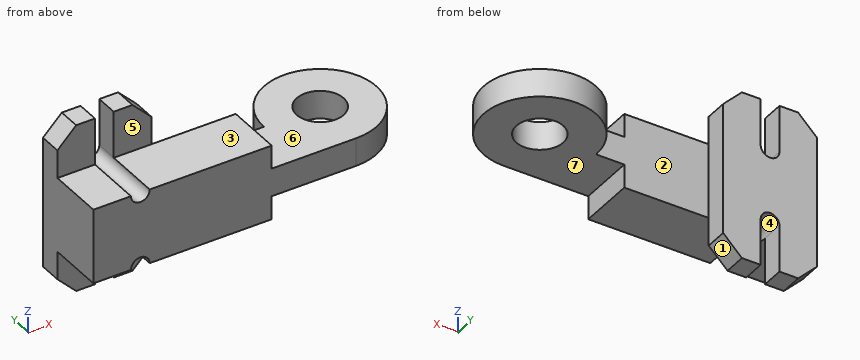
Autodesk Inventor part; units mm, degrees
ref_plane "YZ Plane" through (0, 0, 0) normal (1, 0, 0) x (0, 1, 0)
ref_plane "XZ Plane" through (0, 0, 0) normal (0, 1, 0) x (-1, 0, 0)
ref_plane "XY Plane" through (0, 0, 0) normal (0, 0, 1) x (1, 0, 0)
sketch "Esboço1" plane through (0, 0, 0) normal (0, 0, 1) x (1, 0, 0)
  line L0 (0, 0) -> (95, 0)
  line L1 (95, 0) -> (95, 30)
  line L2 (95, 30) -> (0, 30)
  line L3 (0, 30) -> (0, 0)
  line L4 (0, 30) -> (50, 30)
  line L5 (50, 30) -> (50, 42)
  line L6 (50, 42) -> (0, 42)
  line L7 (0, 42) -> (0, 30)
  line L8 (95, 0) -> (140, 0)
  line L9 (110, 30) -> (95, 30)
  line L10 (95, 30) -> (95, 0)
  arc A0 (140, 0) -> (110, 30) centre (140, 30) ccw
  dimension "d0" = 95
  dimension "d1" = 30
  dimension "d2" = 50
  dimension "d3" = 12
  dimension "d5" = 60
  dimension "d6" = 140
extrude "Extrusão1" add sketch "Esboço1" along normal mid plane 40 contours L3 L2 L1 L0
extrude "Extrusão2" add sketch "Esboço1" along normal mid plane 90 contours L7 L6 L5 L2
extrude "Extrusão3" add sketch "Esboço1" along normal mid plane 15 contours L1 L9 A0 L8
sketch "Esboço2" plane through (0, 0, 7.5) normal (0, 0, 1) x (1, 0, 0)
  arc A0 (140, 0) -> (110, 30) centre (140, 30) ccw
  point P0 (0, 0)
hole "Furo1" at (140, 30, 7.5) direction (0, 0, -1) diameter 25 end through all
sketch "Esboço3" plane through (0, 42, 45) normal (0, 1, 0) x (1, 0, 0)
  line L0 (25, -25) -> (25, 25) construction
  line L1 (50, 0) -> (0, 0)
  line L2 (30, -25) -> (30, 25)
  line L3 (20, 25) -> (20, -25)
  arc A0 (20, -25) -> (30, -25) centre (25, -25) ccw
  arc A1 (30, 25) -> (20, 25) centre (25, 25) ccw
  line L4 (25, 115) -> (25, 65) construction
  line L5 (50, 90) -> (0, 90)
  line L6 (20, 115) -> (20, 65)
  line L7 (30, 65) -> (30, 115)
  arc A2 (30, 115) -> (20, 115) centre (25, 115) ccw
  arc A3 (20, 65) -> (30, 65) centre (25, 65) ccw
  point P0 (0, 45)
  point P1 (25, 0)
  point P2 (25, 90)
  point P3 (20, 0)
  point P4 (30, 0)
  dimension "d20" = 5
  dimension "d21" = 5
  dimension "d22" = 25
  dimension "d23" = 25
extrude "Extrusão4" cut sketch "Esboço3" against normal through all contours L1 L3 A1 L2
extrude "Extrusão5" cut sketch "Esboço3" against normal through all contours L7 A3 L6 L5 | L5 L6 A2 L7
chamfer "Chanfro1" distance 10 angle 45 1 edges at (0, 36, 45) measured on face at (0, 10, 6.6667)
chamfer "Chanfro2" distance 10 angle 45 1 edges at (50, 36, 45) measured on face at (50, 38, -6.6667)
chamfer "Chanfro3" distance 10 angle 45 1 edges at (50, 36, -45) measured on face at (50, 38, -10)
chamfer "Chanfro4" distance 10 angle 45 1 edges at (0, 36, -45) measured on face at (0, 10, 6.6667)
properties part number "Peça teste 4"
Design review of the part built by this model. Coordinates are the model's own, in mm. Face numbers are marked on the shaded views. A direction names the side the tool comes from. Round coordinates to 2 decimals unless told otherwise and drop trailing zeros. Loops run counter-clockwise (first coordinate to the right, second up) from the corner with the lowest first, then second, coordinate; pieces in that order, holes last. Notation, with made-up numbers: (-31.5, 7.25) - (-15.5, 7.25) arc R30 ccw to (-15.5, 29.25) - close; hole circle Ø8 at (78.5, -35). An arc over 180 degrees is marked (long way). One line per item, written item: value. Start each with the question number.
1) Consider section B-B on y = 15. Give the boundary of the cut face in (x, z).
2) For the marked faces 5, 6 and 7, list the 3-axis set-ups (+Z, -Z, +X, -X, +Y, -Y) from which the entire face can be reached by the end or side of a thin tool; tool diameter is ignored.
3) Draft analysis for pull direction X (two halves, no side actions). For the marked faces 1, 2, 3 and 4, state which applies: +X half, -X half, draft (parallel to the pull), parting line (faces both ways), or undercut.
4) To check wall thickness, follow L1, parallel to Y at x = 140, z = 3; L2, parallel to Z at x = 41, y = 3; L3, parallel to Y at x = 8, z = -25. State the ranges of each line that lie inside material, in increasing order. Write a range as from..to.
5) Consider section A-A on x = 33. Give the boundary of the cut face in (y, z).
6) Insertion check: pin 1 Ø2 at (x, y) = (89, 7) entering from -Z; pin 2 Ø12 at (y, z) = (36.5, 28.5) entering from -X; pin 3 Ø16 at (x, z) = (43.5, 38) entering from -Y; pin 4 Ø1 at (y, z) = (20, -19) entering from +X. Each pin has a flat end and moves straight along its axis. Give the tip position at first contact, or say it passes through.
7) Consider section C-C on x = 147. Give the boundary of the cut face in (y, z).
8) Consider section D-D on y = 6.5. Give the boundary of the cut face in (x, z).
Reported:
1. outline: (0, -20) - (20, -20) arc R5 cw to (30, -20) - (95, -20) - (95, -7.5) - (165.98, -7.5) - (165.98, 7.5) - (95, 7.5) - (95, 20) - (30, 20) arc R5 cw to (20, 20) - (0, 20) - close
2. face 5: +Z, +X, -X, -Y
2. face 6: +Z, +X, +Y, -Y
2. face 7: -Z, +X, +Y, -Y
3. face 1: +X half
3. face 2: undercut
3. face 3: draft
3. face 4: undercut
4. L1: y = 0..17.5, 42.5..60
4. L2: z = -20..20
4. L3: y = 30..42
5. outline: (0, -20) - (30, -20) - (30, -45) - (42, -45) - (42, 45) - (30, 45) - (30, 20) - (0, 20) - close
6. pin 1: stops at z = -20
6. pin 2: stops at x = 0
6. pin 3: stops at y = 30
6. pin 4: stops at x = 95
7. outline: (0.83, -7.5) - (19.64, -7.5) - (19.64, 7.5) - (0.83, 7.5) - close; (40.36, -7.5) - (59.17, -7.5) - (59.17, 7.5) - (40.36, 7.5) - close
8. outline: (0, -20) - (20, -20) arc R5 cw to (30, -20) - (95, -20) - (95, -7.5) - (158.65, -7.5) - (158.65, 7.5) - (95, 7.5) - (95, 20) - (30, 20) arc R5 cw to (20, 20) - (0, 20) - close
